```python
from build123d import *

# Parameters (mm, degrees)
SKETCH1_W           = 9
SKETCH1_H           = 9
BOSS_EXTRUDE1_DEPTH = 3
SKETCH2_W           = 2.95
SKETCH2_H           = 6
BOSS_EXTRUDE2_DEPTH = 6.1
FILLET1_R           = 3
SKETCH3_R           = 0.975
CUT_EXTRUDE1_DEPTH  = 11.1
CUT_EXTRUDE3_DEPTH  = 21.1
BOSS_EXTRUDE3_START = 4
SKETCH5_R           = 3
BOSS_EXTRUDE3_DEPTH = 4
SKETCH8_R           = 1.55
CUT_EXTRUDE4_DEPTH  = 5
CUT_EXTRUDE5_DEPTH  = 0.5
BOSS_EXTRUDE4_START = 4
BOSS_EXTRUDE4_DEPTH = 4
BOSS_EXTRUDE5_DEPTH = 0.5
BOSS_EXTRUDE6_DEPTH = 0.5
SKETCH15_W          = 0.501923789
SKETCH15_H          = 0.5
CUT_EXTRUDE6_DEPTH  = 19.5
SKETCH16_R          = 1.45
CUT_EXTRUDE7_DEPTH  = 19.5
FILLET2_R           = 0.5


with BuildPart() as part:
    # Sketch1 → Boss-Extrude1 (new body)
    with BuildSketch(Plane(origin=(0, 0, 0), x_dir=(1, 0, 0), z_dir=(0, 1, 0))):
        with Locations((4.5, 4.5)):
            Rectangle(SKETCH1_W, SKETCH1_H)
    extrude(amount=BOSS_EXTRUDE1_DEPTH)

    # Sketch2 → Boss-Extrude2 (add)
    with BuildSketch(Plane(origin=(0, 0, -9), x_dir=(-1, 0, 0), z_dir=(0, 0, -1))):
        with Locations((-7.525, 1.5)):
            Rectangle(SKETCH2_W, SKETCH2_H)
        with Locations((-1.475, 1.5)):
            Rectangle(SKETCH2_W, SKETCH2_H)
    extrude(amount=BOSS_EXTRUDE2_DEPTH)

    # Fillet1
    fillet1_edges = [part.edges().sort_by_distance(p)[0] for p in [
        (1.475, 4.5, -15.1),
        (1.475, -1.5, -15.1),
        (7.525, -1.5, -15.1),
        (7.525, 4.5, -15.1),
    ]]
    fillet(fillet1_edges, radius=FILLET1_R - 0.0001)  # a hair under: the kernel refuses the full size

    # Sketch3 → Cut-Extrude1 (cut)
    with BuildSketch(Plane(origin=(9, 0, 0), x_dir=(0, 0, -1), z_dir=(1, 0, 0))):
        with Locations((12.1, 1.5)):
            Circle(SKETCH3_R)
    extrude(amount=-CUT_EXTRUDE1_DEPTH, mode=Mode.SUBTRACT)

    # Sketch6 → Cut-Extrude3 (cut)
    with BuildSketch(Plane.ZY):
        with BuildLine():
            Line((-12.1, 4.5), (-9, 4.5))
            Line((-9, 4.5), (-9, 3))
            Line((-9, 3), (-9.501923789, 3))
            ThreePointArc((-9.501923789, 3), (-10.6, 4.098076211), (-12.1, 4.5))
        make_face()
        with BuildLine():
            Line((-12.1, -1.5), (-9, -1.5))
            Line((-9, -1.5), (-9, 0))
            Line((-9, 0), (-9.501923789, 0))
            ThreePointArc((-9.501923789, 0), (-10.6, -1.098076211), (-12.1, -1.5))
        make_face()
    extrude(amount=-CUT_EXTRUDE3_DEPTH, mode=Mode.SUBTRACT)

    # Sketch5 → Boss-Extrude3 (add)
    with BuildSketch(Plane.ZY.offset(BOSS_EXTRUDE3_START)):
        with Locations((-12.1, 1.5)):
            Circle(SKETCH5_R)
    extrude(amount=-BOSS_EXTRUDE3_DEPTH)

    # Sketch8 → Cut-Extrude4 (cut)
    with BuildSketch(Plane(origin=(0, -1.5, 0), x_dir=(-1, 0, 0), z_dir=(0, -1, 0))):
        with Locations(Location((1.6, 12.1, 0), (0, 0, 90))):
            Circle(SKETCH8_R)
    extrude(amount=-CUT_EXTRUDE4_DEPTH, mode=Mode.SUBTRACT)

    # Sketch9 → Cut-Extrude5 (cut)
    with BuildSketch(Plane.ZY.offset(4)):
        with BuildLine():
            Line((-11.85, 1.5), (-11.85, -0.8))
            ThreePointArc((-11.85, -0.8), (-12.1, -1.05), (-12.35, -0.8))
            Line((-12.35, -0.8), (-12.35, 0.896446609))
            Line((-12.35, 0.896446609), (-13.549568901, -0.303122292))
            ThreePointArc((-13.549568901, -0.303122292), (-13.903122292, -0.303122292), (-13.903122292, 0.050431099))
            Line((-13.903122292, 0.050431099), (-12.703553391, 1.25))
            Line((-12.703553391, 1.25), (-14.4, 1.25))
            ThreePointArc((-14.4, 1.25), (-14.65, 1.5), (-14.4, 1.75))
            Line((-14.4, 1.75), (-12.703553391, 1.75))
            Line((-12.703553391, 1.75), (-13.903122292, 2.949568901))
            ThreePointArc((-13.903122292, 2.949568901), (-13.903122292, 3.303122292), (-13.549568901, 3.303122292))
            Line((-13.549568901, 3.303122292), (-12.35, 2.103553391))
            Line((-12.35, 2.103553391), (-12.35, 3.8))
            ThreePointArc((-12.35, 3.8), (-12.1, 4.05), (-11.85, 3.8))
            Line((-11.85, 3.8), (-11.85, 1.5))
        make_face()
    extrude(amount=-CUT_EXTRUDE5_DEPTH, mode=Mode.SUBTRACT)

    # Sketch10 → Boss-Extrude4 (add)
    with BuildSketch(Plane.ZY.offset(BOSS_EXTRUDE4_START)):
        with BuildLine():
            Line((-9.501923789, 0), (0, 0))
            Line((0, 0), (0, 3))
            Line((0, 3), (-9.501923789, 3))
            ThreePointArc((-9.501923789, 3), (-9.1, 1.5), (-9.501923789, 0))
        make_face()
    extrude(amount=-BOSS_EXTRUDE4_DEPTH)

    # Sketch12 → Boss-Extrude5 (add)
    with BuildSketch(Plane.XZ):
        Polygon((9, 0), (-4, 0), (-4, -9.501923789), (2.95, -9.501923789), (2.95, -9), (6.05, -9), (6.05, -9.501923789), (9, -9.501923789), align=None)
    extrude(amount=BOSS_EXTRUDE5_DEPTH)

    # Sketch13 → Boss-Extrude6 (add)
    with BuildSketch(Plane(origin=(0, 3, 0), x_dir=(1, 0, 0), z_dir=(0, 1, 0))):
        Polygon((2.95, 9.501923789), (-4, 9.501923789), (-4, 0), (9, 0), (9, 9.501923789), (6.05, 9.501923789), (6.05, 9), (2.95, 9), align=None)
    extrude(amount=BOSS_EXTRUDE6_DEPTH)

    # Sketch15 → Cut-Extrude6 (cut)
    with BuildSketch(Plane(origin=(9, 0, 0), x_dir=(0, 0, -1), z_dir=(1, 0, 0))):
        with Locations((9.250961895, 3.25)):
            Rectangle(SKETCH15_W, SKETCH15_H)
        with Locations((9.250961895, -0.25)):
            Rectangle(SKETCH15_W, SKETCH15_H)
    extrude(amount=-CUT_EXTRUDE6_DEPTH, mode=Mode.SUBTRACT)

    # Sketch16 → Cut-Extrude7 (cut)
    with BuildSketch(Plane(origin=(0, 3.5, 0), x_dir=(1, 0, 0), z_dir=(0, 1, 0))):
        with Locations(Location((6, 3, 0), (0, 0, 270))):
            Circle(SKETCH16_R)
        with Locations(Location((-1, 3, 0), (0, 0, 90))):
            Circle(SKETCH16_R)
    extrude(amount=-CUT_EXTRUDE7_DEPTH, mode=Mode.SUBTRACT)

    # Fillet2
    fillet2_edges = [part.edges().sort_by_distance(p)[0] for p in [
        (2.5, 3.5, 0),
        (9, 1.25, 0),
        (2.5, -0.5, 0),
        (-4, 1.5, 0),
        (-4, -0.5, -4.5),
        (-4, 3.5, -4.5),
        (9, 3.5, -4.5),
        (9, -0.5, -4.5),
        (2.5, 3.5, -9),
        (2.5, -0.5, -9),
    ]]
    fillet(fillet2_edges, radius=FILLET2_R - 0.0001)  # a hair under: the kernel refuses the full size


solid = part.part
```
The model under review builds one solid part; all positions refer to its coordinate system, in mm. A direction names the side the tool comes from. Give positions to 0.01 mm unless a question says otherwise; leave off trailing zeros. Loops run counter-clockwise (first coordinate to the right, second up) from the corner with the lowest first, then second, coordinate; pieces in that order, holes last. Notation, with made-up numbers: (-29.75, 27) - (-25.75, 27) arc R26 cw to (-25.75, 47) - close; hole circle Ø11 at (-28, 47.5). An arc over 180 degrees is marked (long way). Answer as a JSON object with one key per item and string values.
Q1. Add section C-C on x = 4. State the section outline as (y, z) points, plus the area to 3 significant figures.
Worked out:
{"outline": "(-0.5, -8.5) arc R0.5 ccw to (0, -9) - (3, -9) arc R0.5 ccw to (3.5, -8.5) - (3.5, -0.5) arc R0.5 ccw to (3, 0) - (0, 0) arc R0.5 ccw to (-0.5, -0.5) - close", "area": "35.8 mm^2"}
Q2. Mouldability with a two-part tool opening along Z and no side actions: class faces 1 (the flat face through (2, 3.5, -5)), 2 (the cylindrical face through (7.5, 3.64, -14.2)), 3 (the flat face through (-2, 3.5, -12)) as +Z half, -Z half, draft (parallel to the pull), parting line (faces both ways), or undercut.
Worked out:
{"face 1": "draft", "face 2": "-Z half", "face 3": "undercut"}
Q3. Insertion check: pin 1 (1 mm diameter, centred on x = 3, z = -10.5, fed in from +Y); pin 2 (0.6 mm diameter, centred on y = 2, z = -12, fed in from +X); pin 3 (2.5 mm diameter, centred on x = 2, z = -6, fed in from -Y). Each pin has a flat end and moves straight along its axis. Give the tip position at first contact, or say it passes through.
Worked out:
{"pin 1": "stops at y = 4.29", "pin 2": "stops at x = 0", "pin 3": "stops at y = -0.5"}
Q4. Add section A-A on z = -3. State the section outline as (x, y) points, plus the area to 3 significant figures.
Worked out:
{"outline": "(-4, 0) arc R0.5 ccw to (-3.5, -0.5) - (-2.45, -0.5) - (-2.45, 3.5) - (-3.5, 3.5) arc R0.5 ccw to (-4, 3) - close; (0.45, -0.5) - (4.55, -0.5) - (4.55, 3.5) - (0.45, 3.5) - close; (7.45, -0.5) - (8.5, -0.5) arc R0.5 ccw to (9, 0) - (9, 3) arc R0.5 ccw to (8.5, 3.5) - (7.45, 3.5) - close", "area": "28.6 mm^2"}
Q5. To check wall thickness, follow line 1 along X through (y, z) = (2.3, -3); line 2 along X through (y, z) = (2.75, -12); line 3 along Z through (x, y) = (3.5, 1.75). State the ranges of each line that lie inside material, in increasing order.
Worked out:
{"line 1": "x = -4 to -2.45, 0.45 to 4.55, 7.45 to 9", "line 2": "x = -3.5 to -3.15, -0.05 to 2.95, 6.05 to 9", "line 3": "z = -9 to 0"}
Q6. Add section D-D on z = -9.75. State the section outline as (x, y) points.
Worked out:
{"outline": "(-4, -0.36) - (2.95, -0.36) - (2.95, 3.36) - (-4, 3.36) - close; (6.05, -0.36) - (9, -0.36) - (9, 3.36) - (6.05, 3.36) - close"}
Q7. Add section B-B on y = 2.75. Count the separate pieces of the cut face and the enclosed holes in it, plus the area to 3 significant figures.
Worked out:
{"separate pieces": "1", "enclosed holes": "3", "area": "153 mm^2"}
Q8. For faces 4 (the flat face through (2, -0.5, -4)), 5 (the flat face through (-3.754, 2.341, -13.295)), 6 (the cylindrical face through (7.546, 1.543, -11.126)), 7 (the flat face through (6.05, 1, -11)), 8 (the cylindrical face through (7.5, -1.1, -10.6)), list the 3-axis set-ups (+Z, -Z, +X, -X, +Y, -Y) from which the entire face can be reached by the end or side of a thin tool; tool diameter is ignored.
Worked out:
{"face 4": "+Z, +X, -X, -Y", "face 5": "-X", "face 6": "+X", "face 7": "-Z, +Y, -Y", "face 8": "+X, -X, -Y"}
